Verification items for the finished model (mm, model axes). Face numbers are marked on the shaded views. Round coordinates to 2 decimals unless told otherwise and drop trailing zeros. Order: outer loops, then holes, each group sorted by start corner. A loop starts at its lowest first (then second) coordinate and runs counter-clockwise, first axis right, second up. Notation, with made-up numbers: M 17.5,-0.75 L 67.5,-0.75 A22 ccw 67.5,7.25 Z; hole C -24,43.25 d2. An arc over 180 degrees is marked long. Return JSON: item names as keys, results as strings. Group by question number.
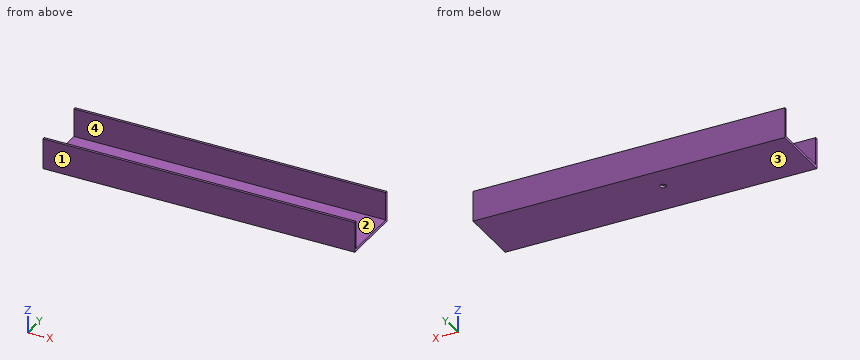
from build123d import *

# Parameters (mm, degrees)
BOSS_EXTRUDE1_DEPTH = 175
SKETCH2_R           = 2.55
CUT_EXTRUDE1_DEPTH  = 380
BOSS_EXTRUDE2_DEPTH = 80


with BuildPart() as part:
    # Sketch1 → Boss-Extrude1 (new body)
    with BuildSketch(Plane(origin=(0, 0, 0), x_dir=(0, 0, -1), z_dir=(1, 0, 0))):
        Polygon((0, 24.377952756), (23, 24.377952756), (23, -21.622047244), (0, -21.622047244), (0, -23.622047244), (25, -23.622047244), (25, 26.377952756), (0, 26.377952756), align=None)
    extrude(amount=BOSS_EXTRUDE1_DEPTH)

    # Sketch2 → Cut-Extrude1 (cut)
    with BuildSketch(Plane(origin=(0, 0, -25), x_dir=(-1, 0, 0), z_dir=(0, 0, -1))):
        with Locations((-30, 6.377952756)):
            Circle(SKETCH2_R)
    extrude(amount=-CUT_EXTRUDE1_DEPTH, mode=Mode.SUBTRACT)

    # Sketch3 → Boss-Extrude2 (add)
    with BuildSketch(Plane.ZY):
        Polygon((0, 26.377952756), (-25, 26.377952756), (-25, -23.622047244), (0, -23.622047244), (0, -21.622047244), (-23, -21.622047244), (-23, 24.377952756), (0, 24.377952756), align=None)
    extrude(amount=BOSS_EXTRUDE2_DEPTH)


solid = part.part
1. Draft check along Y on the marked faces 1, 2, 3 and 4. Enter one of: +Y half, -Y half, draft (parallel to the pull), parting line (faces both ways), or undercut.
2. Cross-section at D-D (y = -16.5). Enter the section's corners in (x, z).
3. Cross-section at C-C (x = 102). Enter the section's corners in (y, z), plus the area to 3 significant figures.
4. Cross-section at B-B (x = 30). Enter the section's corners in (y, z).
5. Go/stop test with a flat-tipped pin: pin 1 (5 mm diameter, centred on x = 126.5, y = -9, fed in from +Z). Record where the tip stops, or that it passes through.
6. Thickness scan on line 1 along Y through (x, z) = (30, -23.55); line 2 along Y through (x, z) = (-0.5, -7.25); line 3 along Z through (x, y) = (68, 4.5). Record the ranges inside material, lowest first. Write a range as from..to.
7. Cross-section at A-A (z = -8.5). Enter the section's corners in (x, y), plus the area to 3 significant figures.
Computed:
{
 "1": {"face 1": "-Y half", "face 2": "undercut", "face 3": "draft", "face 4": "undercut"},
 "2": {"outline": "M -80,-25 L 175,-25 L 175,-23 L -80,-23 Z"},
 "3": {"outline": "M -23.62,-25 L 26.38,-25 L 26.38,0 L 24.38,0 L 24.38,-23 L -21.62,-23 L -21.62,0 L -23.62,0 Z", "area": "192 mm²"},
 "4": {"outline": "M -23.62,-25 L 3.83,-25 L 3.83,-23 L -21.62,-23 L -21.62,0 L -23.62,0 Z; M 8.93,-25 L 26.38,-25 L 26.38,0 L 24.38,0 L 24.38,-23 L 8.93,-23 Z"},
 "5": {"pin 1": "stops at z = -23"},
 "6": {"line 1": "y = -23.62..3.83, 8.93..26.38", "line 2": "y = -23.62..-21.62, 24.38..26.38", "line 3": "z = -25..-23"},
 "7": {"outline": "M -80,-23.62 L 175,-23.62 L 175,-21.62 L -80,-21.62 Z; M -80,24.38 L 175,24.38 L 175,26.38 L -80,26.38 Z", "area": "1,020 mm²"}
}
